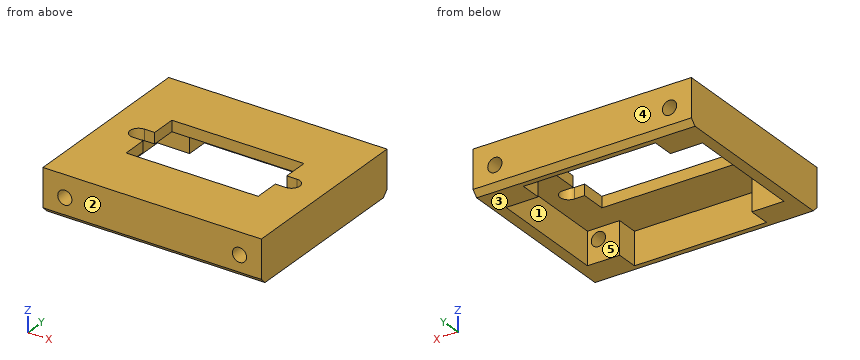
```python
from build123d import *

# Parameters (mm, degrees)
SKETCH_1_W          = 40
SKETCH_1_H          = 34
EXTRUDE_1_DEPTH     = 2
SKETCH_2_W          = 24.2
SKETCH_2_H          = 12.4
CUT_EXTRUDE_1_DEPTH = 2
SKETCH_3_W          = 2
SKETCH_3_H          = 34
EXTRUDE_2_DEPTH     = 6
SKETCH_5_W          = 36
SKETCH_5_H          = 1.98
EXTRUDE_3_DEPTH     = 6
SKETCH_6_W          = 5.9
SKETCH_6_H          = 4
EXTRUDE_4_DEPTH     = 6
SKETCH_7_R          = 1.3
CUT_EXTRUDE_2_DEPTH = 40.899874687
CHAMFER_1_SIZE      = 1


with BuildPart() as part:
    # ｽｹｯﾁ1 → ﾎﾞｽ - 押し出し1 (new body)
    with BuildSketch(Plane.XY):
        Rectangle(SKETCH_1_W, SKETCH_1_H)
    extrude(amount=EXTRUDE_1_DEPTH)

    # ｽｹｯﾁ2 → ｶｯﾄ - 押し出し1 (cut)
    with BuildSketch(Plane.XY.offset(2)):
        Rectangle(SKETCH_2_W, SKETCH_2_H)
        with BuildLine():
            Line((-14, 1.55), (14, 1.55))
            ThreePointArc((14, 1.55), (15.55, 0), (14, -1.55))
            Line((14, -1.55), (-14, -1.55))
            ThreePointArc((-14, -1.55), (-15.55, 0), (-14, 1.55))
        make_face()
    extrude(amount=-CUT_EXTRUDE_1_DEPTH, mode=Mode.SUBTRACT)

    # ｽｹｯﾁ3 → ﾎﾞｽ - 押し出し2 (add)
    with BuildSketch(Plane(origin=(0, 0, 0), x_dir=(-1, 0, 0), z_dir=(0, 0, -1))):
        with Locations((19, 0)):
            Rectangle(SKETCH_3_W, SKETCH_3_H)
        with Locations((-19, 0)):
            Rectangle(SKETCH_3_W, SKETCH_3_H)
    extrude(amount=EXTRUDE_2_DEPTH)

    # ｽｹｯﾁ5 → ﾎﾞｽ - 押し出し3 (add)
    with BuildSketch(Plane(origin=(0, 0, 0), x_dir=(-1, 0, 0), z_dir=(0, 0, -1))):
        with Locations((0, 16.01)):
            Rectangle(SKETCH_5_W, SKETCH_5_H)
        with Locations((0, -16.01)):
            Rectangle(SKETCH_5_W, SKETCH_5_H)
    extrude(amount=EXTRUDE_3_DEPTH)

    # ｽｹｯﾁ6 → ﾎﾞｽ - 押し出し4 (add)
    with BuildSketch(Plane(origin=(0, 0, 0), x_dir=(-1, 0, 0), z_dir=(0, 0, -1))):
        with Locations((-15.05, 13.02)):
            Rectangle(SKETCH_6_W, SKETCH_6_H)
        with Locations((15.05, 13.02)):
            Rectangle(SKETCH_6_W, SKETCH_6_H)
        with Locations((15.05, -13.02)):
            Rectangle(SKETCH_6_W, SKETCH_6_H)
        with Locations((-15.05, -13.02)):
            Rectangle(SKETCH_6_W, SKETCH_6_H)
    extrude(amount=EXTRUDE_4_DEPTH)

    # ｽｹｯﾁ7 → ｶｯﾄ - 押し出し2 (cut, through all)
    with BuildSketch(Plane(origin=(0, 17, 0), x_dir=(1, 0, 0), z_dir=(0, 1, 0))):
        with Locations(Location((-16, 2, 0), (0, 0, 270))):
            Circle(SKETCH_7_R)
        with Locations(Location((16, 2, 0), (0, 0, 270))):
            Circle(SKETCH_7_R)
    extrude(amount=-CUT_EXTRUDE_2_DEPTH, mode=Mode.SUBTRACT)

    # 面取り1
    chamfer_1_edges = [part.edges().sort_by_distance(p)[0] for p in [
        (0, 17, -6),
        (0, -17, -6),
    ]]
    chamfer(chamfer_1_edges, length=CHAMFER_1_SIZE)


solid = part.part
```
Read the model definition and answer for the solid it produces. Units are mm, in the model's axes. Face numbers are marked on the shaded views. A direction names the side the tool comes from. Coordinates: 2 decimals unless noted, no trailing zeros. Write each loop counter-clockwise with the first axis right and the second up, starting at its lowest first coordinate (ties: lowest second). Pieces come first, ordered by that corner, then holes. Notation, with made-up numbers: (-16, 15.25) - (31, 15.25) arc R18 ccw to (31, 50.25) - close; hole circle Ø10 at (70.25, -9). An arc over 180 degrees is marked (long way). Answer as a JSON object with one key per item and string values. Group by question number.
1. A cutting plane is placed at B-B (y = 2.5). Determine the outline of the cut face in (x, z).
2. Which of the six approach directions +Z, -Z, +X, -X, +Y, -Y give full straight-line access (tool end or side, diameter ignored) to the marked faces 4 and 5?
3. The mould has two halves that part along Y. Classify the marked faces 1, 2 and 3: +Y half, -Y half, draft (parallel to the pull), parting line (faces both ways), or undercut.
4. A cutting plane is placed at A-A (x = 16). Determine the outline of the cut face in (y, z).
5. A cutting plane is placed at C-C (z = -2). Give the number of separate pieces and of enclosed holes in the cut face, plus the area to 3 significant figures.
6. A cutting plane is placed at D-D (y = 13.5). Determine the outline of the cut face in (x, z), plus the area to 3 significant figures.
7. Each of these flat-tipped pins is pushed along its axis until it touches: P1, Ø8, axis at x = -11, y = 0.5, coming from the -Z side; P2, Ø4, axis at x = -16, z = -2, coming from the +Y side; P3, Ø4, axis at x = -6, y = -3, coming from the -Z side. Where does it stop, or does it pass through?
8. Consider L1, parallel to X at y = 13.2, z = -2; L2, parallel to X at y = 15.1, z = -2; L3, parallel to Y at x = -10, z = -1.75. Determine where each line is inside the solid, lowest interval first. Write a range as [from, to].
Worked out:
{
 "1": {"outline": "(-20, -6) - (-18, -6) - (-18, 0) - (-12.1, 0) - (-12.1, 2) - (-20, 2) - close; (12.1, 0) - (18, 0) - (18, -6) - (20, -6) - (20, 2) - (12.1, 2) - close"},
 "2": {"face 4": "+Z, -Z, +X, -X, +Y", "face 5": "-Z"},
 "3": {"face 1": "undercut", "face 2": "-Y half", "face 3": "draft"},
 "4": {"outline": "(-17, -5) - (-16, -6) - (-11.02, -6) - (-11.02, -3.3) - (-17, -3.3) - close; (-17, -0.7) - (-11.02, -0.7) - (-11.02, 0) - (11.02, 0) - (11.02, -0.7) - (17, -0.7) - (17, 2) - (-17, 2) - close; (11.02, -6) - (16, -6) - (17, -5) - (17, -3.3) - (11.02, -3.3) - close"},
 "5": {"separate pieces": "4", "enclosed holes": "0", "area": "311 mm²"},
 "6": {"outline": "(-20, -6) - (-12.1, -6) - (-12.1, 0) - (12.1, 0) - (12.1, -6) - (20, -6) - (20, 2) - (-20, 2) - close; hole circle Ø2.6 at (-16, -2); hole circle Ø2.6 at (16, -2)", "area": "164 mm²"},
 "7": {"P1": "stops at z = 0", "P2": "stops at y = 17", "P3": "passes through"},
 "8": {"L1": "x = [-20, -17.3], [-14.7, -12.1], [12.1, 14.7], [17.3, 20]", "L2": "x = [-20, -17.3], [-14.7, 14.7], [17.3, 20]", "L3": "y = [-17, -15.02], [15.02, 17]"}
}
